```python
from build123d import *

# Parameters (mm, degrees)
F0_W     = 90
F0_H     = 20
F1_DEPTH = 10
F3_D     = 2.8
F3_DEPTH = 7
F3_TIP   = 0.8412048666
F5_D     = 2.8
F5_DEPTH = 7
F5_TIP   = 0.8412048666
F6_R     = 3.5
F7_DEPTH = 25


with BuildPart() as f1:
    # F0 (on Top) → F1 (new body)
    with BuildSketch(Plane.XY):
        Rectangle(F0_W, F0_H)
    extrude(amount=F1_DEPTH)

    # F3
    with Locations(Plane(origin=(-45, 0, 0), x_dir=(0, -1, 0), z_dir=(-1, 0, 0))):
        with Locations((-5, 5), (5, 5)):
            Hole(F3_D / 2, depth=F3_DEPTH)
            with Locations((0, 0, -(F3_DEPTH + F3_TIP / 2))):  # 118° drill point
                Cone(0, F3_D / 2, F3_TIP, mode=Mode.SUBTRACT)

    # F5
    with Locations(Plane.YZ.offset(45)):
        with Locations((-5, 5), (5, 5)):
            Hole(F5_D / 2, depth=F5_DEPTH)
            with Locations((0, 0, -(F5_DEPTH + F5_TIP / 2))):  # 118° drill point
                Cone(0, F5_D / 2, F5_TIP, mode=Mode.SUBTRACT)

    # F6 (on face) → F7 (cut)
    with BuildSketch(Plane.XY.offset(10)):
        with Locations((35, 0)):
            Circle(F6_R)
        Circle(F6_R)
        with Locations((-35, 0)):
            Circle(F6_R)
    extrude(amount=-F7_DEPTH, mode=Mode.SUBTRACT)


solid = f1.part
```
Read the model definition and answer for the solid it produces. Units are mm, in the model's axes. A direction names the side the tool comes from. Coordinates: 2 decimals unless noted, no trailing zeros. Order: outer loops, then holes, each group sorted by start corner. A loop starts at its lowest first (then second) coordinate and runs counter-clockwise, first axis right, second up. Notation, with made-up numbers: (-17.75, 43.5) - (13.25, 43.5) arc R23 ccw to (13.25, 68.5) - close; hole circle Ø6 at (29.5, 30.5). An arc over 180 degrees is marked (long way). Answer as a JSON object with one key per item and string values. Group by question number.
Item 1: Section A-A (y = 0) is taken. Give the vertices of the cut face in (x, z), plus the area to 3 significant figures.
Item 2: Section C-C (z = 7.5) is taken. Give the vertices of the cut face in (x, y).
Item 3: Section B-B (x = 35) is taken. Give the vertices of the cut face in (y, z).
Item 4: A tool of negligible diameter and unlimited length cuts with its end or side. For faces 5 (the face through (41.451, -6.335, 5.421)), 6 (the face through (-41.451, 6.335, 5.421)), 7 (the face through (-45, 0, 5)), from which of +Z, -Z, +X, -X, +Y, -Y can it reach the whole face along a straight path? Write none if from no direction.
Item 5: Consider probe 1 along Y at (x, z) = (-41.75, 5); probe 2 along Z at (x, y) = (39.75, -5); probe 3 along Y at (x, z) = (0, 7). Determine where each line is inside the solid, lowest interval first. Write a range as from..to.
Item 6: Flat-ended cylindrical pins translate along their axes: P1, Ø4.5, axis at y = 5, z = 5, coming from the -X side; P2, Ø1.7, axis at y = 5, z = 5, coming from the -X side; P3, Ø5.5, axis at x = 35, y = 0, coming from the -Z side. Find the tip coordinate at first contact, or state that the pin passes through.
Item 7: The mould has two halves that part along Y. Classify faces 1 (the face through (-41.451, -3.665, 5.421)), 2 (the face through (45, 0, 5)), 3 (the face through (-1, -10, 5)), 4 (the face through (32.2, -2.1, 5.1)): +Y half, -Y half, draft (parallel to the pull), parting line (faces both ways), or undercut.
Results are:
{
 "1": {"outline": "(-45, 0) - (-38.5, 0) - (-38.5, 10) - (-45, 10) - close; (-31.5, 0) - (-3.5, 0) - (-3.5, 10) - (-31.5, 10) - close; (3.5, 0) - (31.5, 0) - (31.5, 10) - (3.5, 10) - close; (38.5, 0) - (45, 0) - (45, 10) - (38.5, 10) - close", "area": "690 mm^2"},
 "2": {"outline": "(-45, -10) - (45, -10) - (45, 10) - (-45, 10) - close; hole circle Ø7 at (-35, 0); hole circle Ø7 at (0, 0); hole circle Ø7 at (35, 0)"},
 "3": {"outline": "(-10, 0) - (-3.5, 0) - (-3.5, 10) - (-10, 10) - close; (3.5, 0) - (10, 0) - (10, 10) - (3.5, 10) - close"},
 "4": {"face 5": "+X", "face 6": "-X", "face 7": "+Z, -Z, -X, +Y, -Y"},
 "5": {"probe 1": "y = -10..-6.4, -3.6..3.6, 6.4..10", "probe 2": "z = 0..3.6, 6.4..10", "probe 3": "y = -10..-3.5, 3.5..10"},
 "6": {"P1": "stops at x = -45", "P2": "stops at x = -37.67", "P3": "passes through"},
 "7": {"face 1": "undercut", "face 2": "draft", "face 3": "-Y half", "face 4": "undercut"}
}
